Model file for the job. Use its own axes, mm. A direction names the side the tool comes from. Give positions to 0.01 mm unless a question says otherwise; leave off trailing zeros. Order: outer loops, then holes, each group sorted by start corner. A loop starts at its lowest first (then second) coordinate and runs counter-clockwise, first axis right, second up. Notation, with made-up numbers: (12, -17.5) - (49, -17.5) arc R19 ccw to (49, 11.5) - close; hole circle Ø7 at (29, 62). An arc over 180 degrees is marked (long way). Return JSON: item names as keys, results as strings. Group by question number.
from build123d import *

# Parameters (mm, degrees)
BOSS_EXTRUDE1_DEPTH = 20
SKETCH2_R           = 2.25
CUT_EXTRUDE1_DEPTH  = 79
CUT_EXTRUDE4_DEPTH  = 59
SKETCH7_R           = 2
BOSS_EXTRUDE3_DEPTH = 10
CUT_EXTRUDE5_DEPTH  = 23
BOSS_EXTRUDE2_DEPTH = 20
SKETCH4_R           = 2.25
CUT_EXTRUDE2_DEPTH  = 30
CUT_EXTRUDE6_DEPTH  = 36
SKETCH10_R          = 2
BOSS_EXTRUDE4_DEPTH = 5
SKETCH12_W          = 120
SKETCH12_H          = 5
CUT_EXTRUDE7_DEPTH  = 20


with BuildPart() as part:
    # Sketch1 → Boss-Extrude1 (new body)
    with BuildSketch(Plane.XY):
        with BuildLine():
            Line((-60, 0), (-40, 0))
            ThreePointArc((-40, 0), (-28.284271247, 28.284271247), (0, 40))
            Line((0, 40), (0, 48.461538462))
            Line((0, 48.461538462), (-35.376253193, 48.461538462))
            ThreePointArc((-35.376253193, 48.461538462), (-53.491004812, 27.179264233), (-60, 0))
        make_face()
    boss_extrude1 = extrude(amount=BOSS_EXTRUDE1_DEPTH)

    # Sketch2 → Cut-Extrude1 (cut)
    with BuildSketch(Plane.XZ):
        with Locations((-50, 10)):
            Circle(SKETCH2_R)
    cut_extrude1 = extrude(amount=-CUT_EXTRUDE1_DEPTH, mode=Mode.SUBTRACT)

    # Sketch6 → Cut-Extrude4 (cut)
    with BuildSketch(Plane.XZ):
        with BuildLine():
            Line((-60, 5), (-50, 5))
            ThreePointArc((-50, 5), (-55, 10), (-50, 15))
            Line((-50, 15), (-60, 15))
            Line((-60, 15), (-60, 5))
        make_face()
        with BuildLine():
            ThreePointArc((-50, 15), (-55, 10), (-50, 5))
            Line((-50, 5), (-50, 7.75))
            ThreePointArc((-50, 7.75), (-52.25, 10), (-50, 12.25))
            Line((-50, 12.25), (-50, 15))
        make_face()
        with BuildLine():
            Line((-50, 7.75), (-50, 5))
            ThreePointArc((-50, 5), (-46.464466094, 6.464466094), (-45, 10))
            ThreePointArc((-45, 10), (-46.464466094, 13.535533906), (-50, 15))
            Line((-50, 15), (-50, 12.25))
            ThreePointArc((-50, 12.25), (-48.409009742, 11.590990258), (-47.75, 10))
            ThreePointArc((-47.75, 10), (-48.409009742, 8.409009742), (-50, 7.75))
        make_face()
    cut_extrude4 = extrude(amount=-CUT_EXTRUDE4_DEPTH, mode=Mode.SUBTRACT)

    # Sketch7 → Boss-Extrude3 (add)
    with BuildSketch(Plane.XZ):
        with BuildLine():
            Line((-50, 15), (-60, 15))
            Line((-60, 15), (-60, 5))
            Line((-60, 5), (-50, 5))
            ThreePointArc((-50, 5), (-45, 10), (-50, 15))
        make_face()
        with Locations((-50, 10)):
            Circle(SKETCH7_R, mode=Mode.SUBTRACT)
    boss_extrude3 = extrude(amount=-BOSS_EXTRUDE3_DEPTH)

    # Sketch8 → Cut-Extrude5 (cut)
    with BuildSketch(Plane.XY.offset(20)):
        with BuildLine():
            Line((-64.996039314, 0), (-60, 0))
            ThreePointArc((-60, 0), (-59.578019695, 7.10348993), (-58.31801436, 14.107062099))
            Line((-58.31801436, 14.107062099), (-63.173999234, 15.28171938))
            ThreePointArc((-63.173999234, 15.28171938), (-64.538921839, 7.694978513), (-64.996039314, 0))
        make_face()
    cut_extrude5 = extrude(amount=-CUT_EXTRUDE5_DEPTH, mode=Mode.SUBTRACT)

    # Mirror1: Boss-Extrude1, Cut-Extrude1, Cut-Extrude4, Boss-Extrude3, Cut-Extrude5 across plane
    add(boss_extrude1.mirror(Plane(origin=(0, 0, 20), x_dir=(0, 0, 1), z_dir=(1, 0, 0))))
    add(cut_extrude1.mirror(Plane(origin=(0, 0, 20), x_dir=(0, 0, 1), z_dir=(1, 0, 0))), mode=Mode.SUBTRACT)
    add(cut_extrude4.mirror(Plane(origin=(0, 0, 20), x_dir=(0, 0, 1), z_dir=(1, 0, 0))), mode=Mode.SUBTRACT)
    add(boss_extrude3.mirror(Plane(origin=(0, 0, 20), x_dir=(0, 0, 1), z_dir=(1, 0, 0))))
    add(cut_extrude5.mirror(Plane(origin=(0, 0, 20), x_dir=(0, 0, 1), z_dir=(1, 0, 0))), mode=Mode.SUBTRACT)

    # Sketch3 → Boss-Extrude2 (add)
    with BuildSketch(Plane(origin=(0, 0, 0), x_dir=(-1, 0, 0), z_dir=(0, 0, -1))):
        with BuildLine():
            add(Edge.make_bspline(
                [(-5.376253193, 48.461538462), (2.596156859, 48.461538462), (7.056491998, 53.461538462)],
                knots=[4.71238898, 4.71238898, 4.71238898, 5.689437437, 5.689437437, 5.689437437], degree=2, weights=[1, 0.883026434, 1]))
            Line((-5.376253193, 48.461538462), (35.376253193, 48.461538462))
            ThreePointArc((35.376253193, 48.461538462), (36.710520922, 47.458799538), (38.016381278, 46.419335998))
            Line((38.016381278, 46.419335998), (38.016381278, 53.461538462))
            Line((38.016381278, 53.461538462), (7.056491998, 53.461538462))
        make_face()
    extrude(amount=-BOSS_EXTRUDE2_DEPTH)

    # Sketch4 → Cut-Extrude2 (cut)
    with BuildSketch(Plane(origin=(0, 53.461538462, 0), x_dir=(1, 0, 0), z_dir=(0, 1, 0))):
        with Locations((-29.623746807, -10)):
            Circle(SKETCH4_R)
        with Locations((-14.623746807, -10)):
            Circle(SKETCH4_R)
    extrude(amount=-CUT_EXTRUDE2_DEPTH, mode=Mode.SUBTRACT)

    # Sketch9 → Cut-Extrude6 (cut)
    with BuildSketch(Plane(origin=(0, 53.461538462, 0), x_dir=(1, 0, 0), z_dir=(0, 1, 0))):
        with BuildLine():
            Line((-29.623746807, -5), (-14.623746807, -5))
            ThreePointArc((-14.623746807, -5), (-9.623746807, -10), (-14.623746807, -15))
            Line((-14.623746807, -15), (-29.623746807, -15))
            ThreePointArc((-29.623746807, -15), (-34.623746807, -10), (-29.623746807, -5))
        make_face()
    extrude(amount=-CUT_EXTRUDE6_DEPTH, mode=Mode.SUBTRACT)

    # Sketch10 → Boss-Extrude4 (add)
    with BuildSketch(Plane(origin=(0, 53.461538462, 0), x_dir=(1, 0, 0), z_dir=(0, 1, 0))):
        with BuildLine():
            Line((-29.623746807, -5), (-14.623746807, -5))
            ThreePointArc((-14.623746807, -5), (-9.623746807, -10), (-14.623746807, -15))
            Line((-14.623746807, -15), (-29.623746807, -15))
            ThreePointArc((-29.623746807, -15), (-34.623746807, -10), (-29.623746807, -5))
        make_face()
        with Locations((-29.623746807, -10)):
            Circle(SKETCH10_R, mode=Mode.SUBTRACT)
        with Locations((-14.623746807, -10)):
            Circle(SKETCH10_R, mode=Mode.SUBTRACT)
    extrude(amount=-BOSS_EXTRUDE4_DEPTH)

    # Sketch12 → Cut-Extrude7 (cut)
    with BuildSketch(Plane(origin=(0, 0, 0), x_dir=(-1, 0, 0), z_dir=(0, 0, -1))):
        with Locations((0, 2.5)):
            Rectangle(SKETCH12_W, SKETCH12_H)
    extrude(amount=-CUT_EXTRUDE7_DEPTH, mode=Mode.SUBTRACT)


solid = part.part
(1) Drill centre lines: L1, parallel to Z at x = -55, y = 20.5; L2, parallel to X at y = 36.5, z = 9.5; L3, parallel to X at y = 50.5, z = 10. Where is each one in solid material? Low to high.
(2) Slice it at C-C (y = 29). Give the cut face in (x, z), and give its area (3 significant figures).
(3) Drop flat-ended pins along their axis: pin 1 Ø3 at (x, z) = (-54, 9.5) entering from +Y; pin 2 Ø3.5 at (x, z) = (50, 10) entering from +Y; pin 3 Ø5 at (y, z) = (48.5, 10) entering from -X; pin 4 Ø10 at (x, z) = (16.5, 6) entering from +Y. Give the stop position or say it passes through.
(4) Pull direction X, two halves, no side cores. Call faces 4 (the face through (-9.625, 42.925, 9.89)), 5 (the face through (-22, 48.462, 10)), 6 (the face through (-52.95, 28.22, 3.19)), 7 (the face through (52.134, 29.7, 3.193)): released by +X, released by -X, zero draft, split by the parting line, or undercut.
(5) Slice it at A-A (y = 21.5). Give the cut face in (x, z), and give its area (3 significant figures).
(6) Slice it at B-B (y = 34.5). Give the cut face in (x, z), and give its area (3 significant figures).
(7) 3-axis set-ups, long thin cutter, end or side, ignore diameter. For faces 1 (the face through (-34.623, 34.445, 10.11)), 2 (the face through (52.2, 10, 10.1)), 3 (the face through (20, 48.462, 10)): which of +Z, -Z, +X, -X, +Y, -Y reach the whole face in a straight line?
Result set:
{
 "1": {"L1": "z = 0 to 5, 15 to 20", "L2": "x = -45.03 to -34.6, 16.36 to 45.03", "L3": "x = -38.02 to -31.62, -27.62 to -16.62, -12.62 to -3.2"},
 "2": {"outline": "(-52.53, 0) - (-27.55, 0) - (-27.55, 5) - (-29.62, 5) arc R5 cw to (-29.62, 15) - (-27.55, 15) - (-27.55, 20) - (-52.53, 20) - (-52.53, 15) - (-50, 15) arc R5 cw to (-50, 5) - (-52.53, 5) - close; (27.55, 0) - (52.53, 0) - (52.53, 5) - (50, 5) arc R5 cw to (50, 15) - (52.53, 15) - (52.53, 20) - (27.55, 20) - close", "area": "810 mm²"},
 "3": {"pin 1": "stops at y = 10", "pin 2": "passes through", "pin 3": "stops at x = -38.52", "pin 4": "stops at y = 48.46"},
 "4": {"face 4": "undercut", "face 5": "undercut", "face 6": "released by -X", "face 7": "released by +X"},
 "5": {"outline": "(-56.02, 0) - (-33.73, 0) - (-33.73, 7.15) arc R5 cw to (-33.73, 12.85) - (-33.73, 20) - (-56.02, 20) - (-56.02, 15) - (-50, 15) arc R5 cw to (-50, 5) - (-56.02, 5) - close; (33.73, 0) - (56.02, 0) - (56.02, 5) - (50, 5) arc R5 cw to (50, 15) - (56.02, 15) - (56.02, 20) - (33.73, 20) - close", "area": "689 mm²"},
 "6": {"outline": "(-49.09, 0) - (-20.24, 0) - (-20.24, 5) - (-29.62, 5) arc R5 cw to (-29.62, 15) - (-20.24, 15) - (-20.24, 20) - (-49.09, 20) - (-49.09, 14.92) arc R5 cw to (-49.09, 5.08) - close; (20.24, 0) - (49.09, 0) - (49.09, 5.08) arc R5 cw to (49.09, 14.92) - (49.09, 20) - (20.24, 20) - close", "area": "960 mm²"},
 "7": {"face 1": "-Y", "face 2": "+X, +Y", "face 3": "+Z, -Z, +X, +Y"}
}
